from build123d import *

# Parameters (mm, degrees)
SKETCH1_W                       = 93
SKETCH1_H                       = 80
BOSS_EXTRUDE1_DEPTH             = 1.5
F_5_0MM_PRESS_DOWEL_HOLE1_D     = 5
F_5_0MM_PRESS_DOWEL_HOLE1_DEPTH = 6
F_5_0MM_PRESS_DOWEL_HOLE1_TIP   = 1.502151548
F_3_0MM_DOWEL_HOLE1_D           = 3
F_3_0MM_DOWEL_HOLE2_D           = 3
F_3_0MM_DOWEL_HOLE2_DEPTH       = 2.999
F_3_0MM_DOWEL_HOLE2_TIP         = 0.901290929
F_3_0MM_DOWEL_HOLE3_D           = 3


with BuildPart() as part:
    # Sketch1 → Boss-Extrude1 (new body)
    with BuildSketch(Plane.XY):
        with Locations((46.5, 40)):
            Rectangle(SKETCH1_W, SKETCH1_H)
    extrude(amount=BOSS_EXTRUDE1_DEPTH)

    # Ø5.0mm Press Dowel Hole1
    with Locations(Plane(origin=(19.881275608, -7.745569698, 0), x_dir=(-1, 0, 0), z_dir=(0, 0, -1))):
        with Locations((-15.118724392, 12.745569698), (14.881275608, 12.745569698)):
            Hole(F_5_0MM_PRESS_DOWEL_HOLE1_D / 2, depth=F_5_0MM_PRESS_DOWEL_HOLE1_DEPTH)
            with Locations((0, 0, -(F_5_0MM_PRESS_DOWEL_HOLE1_DEPTH + F_5_0MM_PRESS_DOWEL_HOLE1_TIP / 2))):  # 118° drill point
                Cone(0, F_5_0MM_PRESS_DOWEL_HOLE1_D / 2, F_5_0MM_PRESS_DOWEL_HOLE1_TIP, mode=Mode.SUBTRACT)

    # Ø3.0mm Dowel Hole1 (through all)
    with Locations(Plane(origin=(19.881275608, -7.745569698, -1.5), x_dir=(-1, 0, 0), z_dir=(0, 0, -1))):
        with Locations((-26.893032931, 71.71065686), (-14.67702886, 67.264394997)):
            Hole(F_3_0MM_DOWEL_HOLE1_D / 2)

    # Ø3.0mm Dowel Hole2
    with Locations(Plane(origin=(19.881275608, -7.745569698, 0), x_dir=(-1, 0, 0), z_dir=(0, 0, -1))):
        with Locations((-58.118724392, 67.745569698), (-58.118724392, 47.745569698)):
            Hole(F_3_0MM_DOWEL_HOLE2_D / 2, depth=F_3_0MM_DOWEL_HOLE2_DEPTH)
            with Locations((0, 0, -(F_3_0MM_DOWEL_HOLE2_DEPTH + F_3_0MM_DOWEL_HOLE2_TIP / 2))):  # 118° drill point
                Cone(0, F_3_0MM_DOWEL_HOLE2_D / 2, F_3_0MM_DOWEL_HOLE2_TIP, mode=Mode.SUBTRACT)

    # Ø3.0mm Dowel Hole3 (through all)
    with Locations(Plane(origin=(19.881275608, -7.745569698, 3), x_dir=(1, 0, 0), z_dir=(0, 0, 1))):
        with Locations((-0.881275608, 12.745569698)):
            Hole(F_3_0MM_DOWEL_HOLE3_D / 2)


solid = part.part
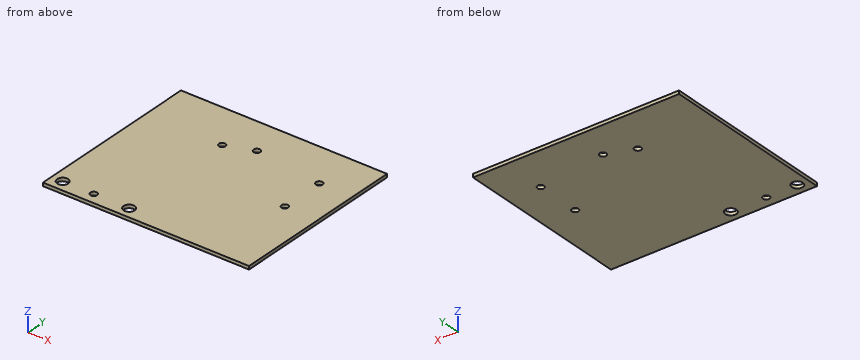
Read the model definition and answer for the solid it produces. Units are mm, in the model's axes. Give positions to 0.01 mm unless a question says otherwise; leave off trailing zeros. Write each loop counter-clockwise with the first axis right and the second up, starting at its lowest first coordinate (ties: lowest second). Pieces come first, ordered by that corner, then holes. Notation, with made-up numbers: (22, 10) - (79, 10) arc R20 ccw to (79, 39) - close; hole circle Ø4 at (52.25, -4). An arc over 180 degrees is marked (long way). Answer in a Markdown table with one row per item. Add a question column.
Item 1: Section D-D, the plane x = 35 is taken. Write down the section's boundary in (y, z).
Item 2: Find the intervals of material crossed by L1, parallel to Y at x = 78, z = 0.3; L2, parallel to Y at x = 35, z = 0.75; L3, parallel to Y at x = 5, z = 0.55, in increasing order.
Item 3: Section B-B, the plane y = 40 is taken. Write down the section's boundary in (x, z).
Item 4: Section A-A, the plane y = 5 is taken. Write down the section's boundary in (x, z), and give its area (3 significant figures).
Item 5: Flat-ended cylindrical pins translate along their axes: P1, Ø2.5, axis at x = 19, y = 5, coming from the +Z side; P2, Ø3.5, axis at x = 78, y = 60, coming from the -Z side. Find the tip coordinate at first contact, or state that the pin passes through.
Item 6: Section C-C, the plane x = 5 is taken. Write down the section's boundary in (y, z).
Recorded:
| question | item | result |
|---|---|---|
| 1 | outline | (0, 0) - (2.5, 0) - (2.5, 1.5) - (0, 1.5) - close; (7.5, 0) - (58.09, 0) - (58.09, 1.5) - (7.5, 1.5) - close; (60.95, 0) - (80, 0) - (80, 1.5) - (60.95, 1.5) - close |
| 2 | L1 | y = 0 to 38.5, 41.5 to 58.5, 61.5 to 80 |
| 2 | L2 | y = 0 to 2.5, 7.5 to 58.09, 60.95 to 80 |
| 2 | L3 | y = 0 to 2.5, 7.5 to 80 |
| 3 | outline | (0, 0) - (76.5, 0) - (76.5, 1.5) - (0, 1.5) - close; (79.5, 0) - (93, 0) - (93, 1.5) - (79.5, 1.5) - close |
| 4 | outline | (0, 0) - (2.5, 0) - (2.5, 1.5) - (0, 1.5) - close; (7.5, 0) - (17.5, 0) - (17.5, 1.5) - (7.5, 1.5) - close; (20.5, 0) - (32.5, 0) - (32.5, 1.5) - (20.5, 1.5) - close; (37.5, 0) - (93, 0) - (93, 1.5) - (37.5, 1.5) - close |
| 4 | area | 120 mm2 |
| 5 | P1 | passes through |
| 5 | P2 | stops at z = 0 |
| 6 | outline | (0, 0) - (2.5, 0) - (2.5, 1.5) - (0, 1.5) - close; (7.5, 0) - (80, 0) - (80, 1.5) - (7.5, 1.5) - close |
